from build123d import *

# Parameters (mm, degrees)
SKETCH6_R               = 10
BOSS_EXTRUDE4_DEPTH     = 2.5
SKETCH7_R               = 6
BOSS_EXTRUDE5_DEPTH     = 6.4
SKETCH8_R               = 6
BOSS_EXTRUDE6_DEPTH     = 6.4
SKETCH12_R              = 10
BOSS_EXTRUDE8_DEPTH     = 5
CUT_EXTRUDE1_DEPTH      = 7.4
CUT_EXTRUDE1_DEPTH_BACK = 17.4


with BuildPart() as part:
    # Sketch6 → Boss-Extrude4 (new body, symmetric)
    with BuildSketch(Plane.XY):
        Circle(SKETCH6_R)
    extrude(amount=BOSS_EXTRUDE4_DEPTH, both=True)

    # Sketch7 → Boss-Extrude5 (add)
    with BuildSketch(Plane.XY.offset(2.5)):
        with Locations((0, 1)):
            Circle(SKETCH7_R)
    extrude(amount=BOSS_EXTRUDE5_DEPTH)

    # Sketch8 → Boss-Extrude6 (add)
    with BuildSketch(Plane(origin=(0, 0, -2.5), x_dir=(-1, 0, 0), z_dir=(0, 0, -1))):
        with Locations((0, -1)):
            Circle(SKETCH8_R)
    extrude(amount=BOSS_EXTRUDE6_DEPTH)

    # Sketch12 → Boss-Extrude8 (add)
    with BuildSketch(Plane(origin=(0, 0, -8.9), x_dir=(-1, 0, 0), z_dir=(0, 0, -1))):
        Circle(SKETCH12_R)
    extrude(amount=BOSS_EXTRUDE8_DEPTH)

    # Sketch11 → Cut-Extrude1 (cut, two sides)
    with BuildSketch(Plane.XY.offset(2.5)) as cut_extrude1_sk:
        with BuildLine():
            Line((-1.774823935, -2.9), (1.774823935, -2.9))
            ThreePointArc((1.774823935, -2.9), (3.4, 0), (1.774823935, 2.9))
            Line((1.774823935, 2.9), (-1.774823935, 2.9))
            ThreePointArc((-1.774823935, 2.9), (-3.4, 0), (-1.774823935, -2.9))
        make_face()
    extrude(amount=CUT_EXTRUDE1_DEPTH, mode=Mode.SUBTRACT)
    extrude(cut_extrude1_sk.sketch, amount=-CUT_EXTRUDE1_DEPTH_BACK, mode=Mode.SUBTRACT)


solid = part.part
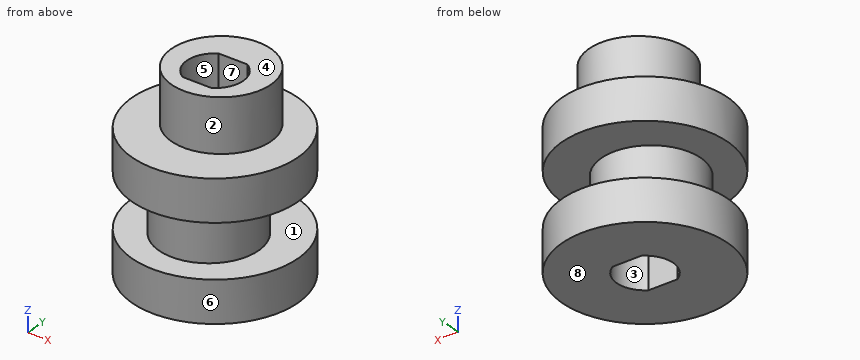
Could you check a few things on this model? Use its own coordinates, in mm. Face numbers are marked on the shaded views. A direction names the side the tool comes from. Give positions to 0.01 mm unless a question says otherwise; leave off trailing zeros. Write each loop counter-clockwise with the first axis right and the second up, starting at its lowest first coordinate (ties: lowest second). Pieces come first, ordered by that corner, then holes. Notation, with made-up numbers: (33.5, 68.25) -> (69.5, 68.25) arc R27 ccw to (69.5, 93.25) -> close; hole circle Ø3 at (-21, -20). An arc over 180 degrees is marked (long way). Answer as a JSON object with one key per item and string values.
Q1. Suppose I cut it at A-A on x = 0. Write out the boundary of the cut face in (y, z), then the cut area to 3 significant figures.
Taken from the geometry:
{"outline": "(-10, -13.9) -> (-2.9, -13.9) -> (-2.9, 8.9) -> (-5, 8.9) -> (-5, 2.5) -> (-10, 2.5) -> (-10, -2.5) -> (-7, -2.5) -> (-7, -8.9) -> (-10, -8.9) -> close; (2.9, -13.9) -> (10, -13.9) -> (10, -8.9) -> (5, -8.9) -> (5, -2.5) -> (10, -2.5) -> (10, 2.5) -> (7, 2.5) -> (7, 8.9) -> (2.9, 8.9) -> close", "area": "221 mm²"}
Q2. Will these pins go through, and if not, where does the flat tip stop? pin 1 Ø3 at (x, z) = (6, 1.5) entering from +Y; pin 2 Ø4 at (y, z) = (3.5, -7) entering from +X; pin 3 Ø1.5 at (y, z) = (-3, 6.5) entering from +X.
Taken from the geometry:
{"pin 1": "stops at y = 8.93", "pin 2": "stops at x = 9.58", "pin 3": "stops at x = 5.04"}
Q3. Please list where these lines run through material, in increasing order: L1, parallel to Z at x = -0.5, y = -8.5; L2, parallel to Z at x = 2, y = 6; L3, parallel to Z at x = -2.25, y = -5.
Taken from the geometry:
{"L1": "z = -13.9 to -8.9, -2.5 to 2.5", "L2": "z = -13.9 to -8.9, -2.5 to 8.9", "L3": "z = -13.9 to 2.5"}
Q4. Which directions (+Z, -Z, +X, -X, +Y, -Y) give clear straight access to the entire face, cutting with the end or side of a thin tool? Please do the marked faces 1, 2, 3 and 4.
Taken from the geometry:
{"face 1": "none", "face 2": "+Z", "face 3": "+Z, -Z", "face 4": "+Z, +X, -X, +Y, -Y"}
Q5. Suppose I cut it at B-B on y = 8. Write out the boundary of the cut face in (x, z).
Taken from the geometry:
{"outline": "(-6, -13.9) -> (6, -13.9) -> (6, -8.9) -> (-6, -8.9) -> close; (-6, -2.5) -> (6, -2.5) -> (6, 2.5) -> (-6, 2.5) -> close"}
Q6. Suppose I cut it at D-D on z = -5.25. Write out the boundary of the cut face in (x, y), then the cut area to 3 significant figures.
Taken from the geometry:
{"outline": "circle Ø12 at (0, -1); hole (-1.77, -2.9) -> (1.77, -2.9) arc R3.4 ccw to (1.77, 2.9) -> (-1.77, 2.9) arc R3.4 ccw to start", "area": "79.2 mm²"}
Q7. We'd pull the mould along X, two halves only. Please class the marked faces 5, 6, 7 and 8: released by +X, released by -X, zero draft, split by the parting line, or undercut.
Taken from the geometry:
{"face 5": "undercut", "face 6": "split by the parting line", "face 7": "undercut", "face 8": "zero draft"}
